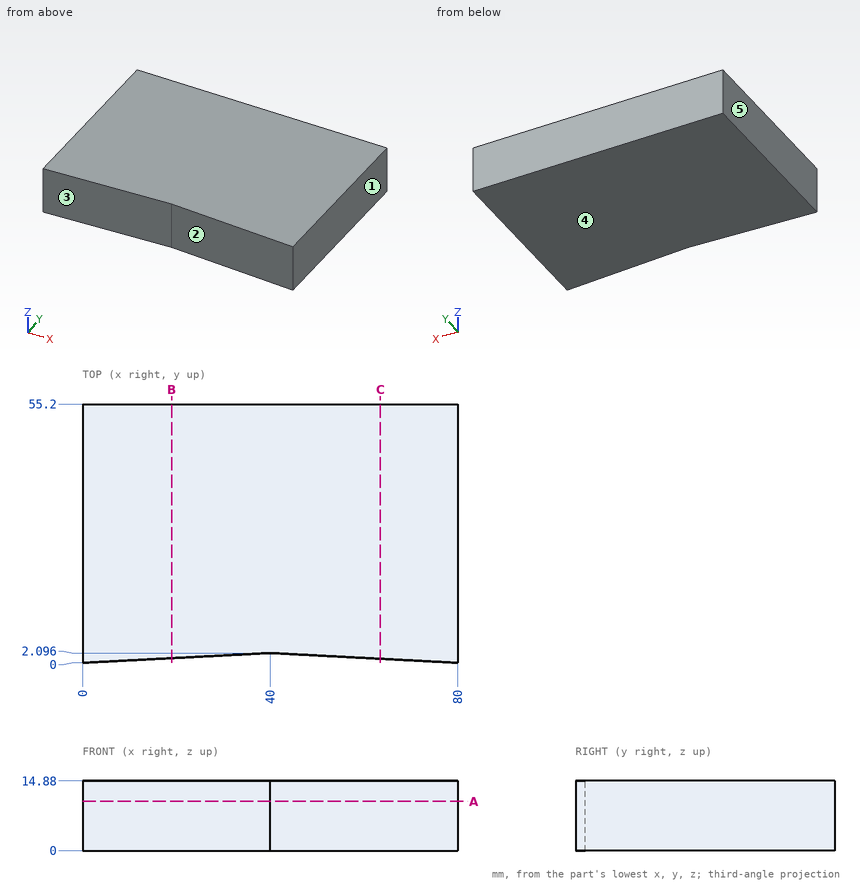
Job drawing, mm, ordinate dimensions from the low corner. One solid piece. A direction names the side the tool comes from. Round coordinates to 2 decimals unless told otherwise and drop trailing zeros. Order: outer loops, then holes, each group sorted by start corner. A loop starts at its lowest first (then second) coordinate and runs counter-clockwise, first axis right, second up. Notation, with made-up numbers: M 7,66.5 L 65,66.5 A5 cw 65,75.5 Z; hole C -26.75,-24 d11. An arc over 180 degrees is marked long. Write each question's results on one line, items separated by ' | '. Start each with the question number.
(1) Probe probe 1 along Y at (x, z) = (36.5, 6.75); probe 2 along Y at (x, z) = (61, 10.5). List the from-to ranges inside material, lowest first. Write a range as from..to.
(2) Saw through at B-B, the plane x = 19. Give the cut face in (y, z).
(3) Saw through at A-A, the plane z = 10.5. Give the cut face in (x, y).
(4) Which spindle directions (+Z, -Z, +X, -X, +Y, -Y) get a long thin tool onto all of the face, cutting with end or side? Do the marked faces 1 and 2. Say none if no direction does.
(5) Saw through at C-C, the plane x = 63.5. Give the cut face in (y, z) (1 decimal).
(6) Two-plate mould, pull along X, no slides. Class the marked faces 3, 4 and 5: pulls with the +X half, pulls with the -X half, needs draft (parallel to the pull), parting line crosses it, or undercut.
Established:
1) probe 1: y = 1.91..55.2 | probe 2: y = 1..55.2
2) outline: M 1,0 L 55.2,0 L 55.2,14.88 L 1,14.88 Z
3) outline: M 0,0 L 40,2.1 L 80,0 L 80,55.2 L 0,55.2 Z
4) face 1: +Z, -Z, +X, +Y, -Y | face 2: +Z, -Z, -Y
5) outline: M 0.9,0 L 55.2,0 L 55.2,14.9 L 0.9,14.9 Z
6) face 3: undercut | face 4: needs draft | face 5: pulls with the -X half
